Verification items for this drawing (mm, ordinates from the low corner). Round coordinates to 2 decimals unless told otherwise and drop trailing zeros. Loops run counter-clockwise (first coordinate to the right, second up) from the corner with the lowest first, then second, coordinate; pieces in that order, holes last. Notation, with made-up numbers: M 40,76 L 49,76 A25 cw 49,96 Z; hole C 83.25,55 d11. An arc over 180 degrees is marked long. Use one line per item in the form item = value. Start each with the question number.
1. Go/stop test with a flat-tipped pin: pin 1 (2 mm diameter, centred on x = 24, y = 8, fed in from -Z). Record where the tip stops, or that it passes through.
2. Cross-section at C-C (y = 5). Record the boundary of the cut face in (x, z), then the cut area to 3 significant figures.
3. Draft check along Y on the marked faces 1, 2 and 3. Enter one of: pulls with the +Y half, pulls with the -Y half, needs draft (parallel to the pull), parting line crosses it, or undercut.
4. Material ranges on line 1 (Y direction, x = 25, z = 6.75); line 2 (X direction, y = 5, z = 3.25); line 3 (X direction, y = 5, z = 6), recorded low to high.
5. Cross-section at B-B (x = 5). Record the boundary of the cut face in (y, z), then the cut area to 3 significant figures.
6. Cross-section at A-A (z = 7). Record the boundary of the cut face in (x, y), then the cut area to 3 significant figures.
7. Cross-section at D-D (z = 4). Record the boundary of the cut face in (x, y).
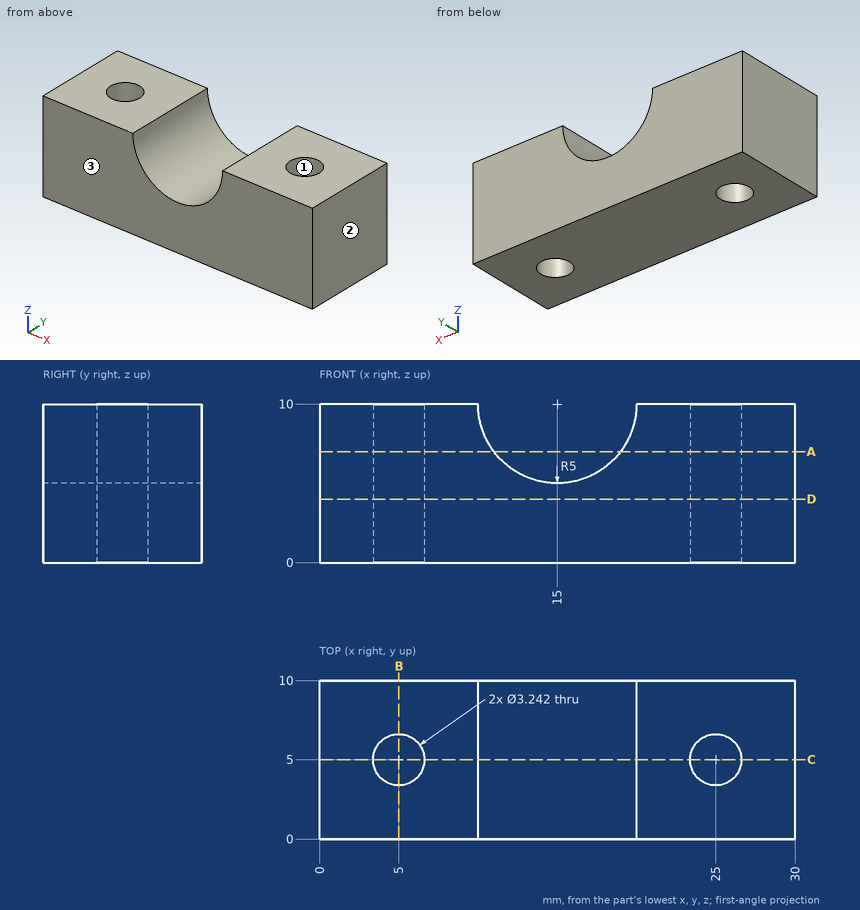
Reported:
q1.pin_1 = 0
q2.outline = M 0,0 L 3.38,0 L 3.38,10 L 0,10 Z; M 6.62,0 L 23.38,0 L 23.38,10 L 20,10 A5 cw 10,10 L 6.62,10 Z; M 26.62,0 L 30,0 L 30,10 L 26.62,10 Z
q2.area = 196 mm²
q3.face_1 = undercut
q3.face_2 = needs draft
q3.face_3 = pulls with the -Y half
q4.line_1 = 0 to 3.38, 6.62 to 10
q4.line_2 = 0 to 3.38, 6.62 to 23.38, 26.62 to 30
q4.line_3 = 0 to 3.38, 6.62 to 12, 18 to 23.38, 26.62 to 30
q5.outline = M 0,0 L 3.38,0 L 3.38,10 L 0,10 Z; M 6.62,0 L 10,0 L 10,10 L 6.62,10 Z
q5.area = 67.6 mm²
q6.outline = M 0,0 L 11,0 L 11,10 L 0,10 Z; M 19,0 L 30,0 L 30,10 L 19,10 Z; hole C 5,5 d3.24; hole C 25,5 d3.24
q6.area = 203 mm²
q7.outline = M 0,0 L 30,0 L 30,10 L 0,10 Z; hole C 5,5 d3.24; hole C 25,5 d3.24
